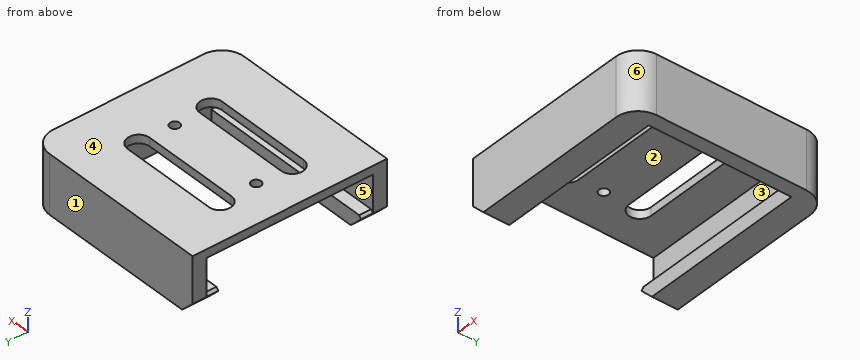
Autodesk Fusion 360 part; units mm, degrees
sketch "Sketch1" plane through (0, 0, 0) normal (0, 0, 1) x (1, 0, 0)
  line L0 (30, 25.7) -> (-30, 25.7)
  line L1 (-30, 25.7) -> (-30, -25.7)
  line L2 (-30, -25.7) -> (30, -25.7)
  line L3 (30, -25.7) -> (30, 25.7)
  line L4 (30, -30) -> (-30, -30)
  line L5 (-30, -35) -> (-30, 35)
  line L6 (-30, 30) -> (30, 30)
  line L7 (30, 30) -> (30, -30)
  line L8 (-30, 35) -> (27, 35)
  line L9 (35, 27) -> (35, -27)
  line L10 (-30, -35) -> (27, -35)
  arc A0 (35, 27) -> (27, 35) centre (27, 27) ccw
  arc A1 (27, -35) -> (35, -27) centre (27, -27) ccw
  circle A2 centre (-20, 0) radius 1.75
  circle A3 centre (15, 0) radius 1.75
  line L11 (-20, 9) -> (15, 9)
  arc A4 (15, 9) -> (15, 17) centre (15, 13) ccw
  line L12 (15, 17) -> (-20, 17)
  arc A5 (-20, 17) -> (-20, 9) centre (-20, 13) ccw
  line L13 (-20, 13) -> (15, 13) construction
  line L14 (1.75, 0) -> (22.5, 0)
  line L15 (-20, -9) -> (15, -9)
  arc A6 (-20, -9) -> (-20, -17) centre (-20, -13) ccw
  line L16 (15, -17) -> (-20, -17)
  arc A7 (15, -17) -> (15, -9) centre (15, -13) ccw
  dimension "d1" = 60
  dimension "d2" = 51.4
  dimension "d3" = 60
  dimension "d6" = 8
  dimension "d15" = 3.5
  dimension "d16" = 3.5
extrude "Extrude1" add sketch "Sketch1" along normal blind 5.5 contours L3 L4 L5 L6 L7 L8 L9 L10 A0 A1 | L0 L5 L6 L7 | L2 L4 L5 L7
extrude "Extrude2" add sketch "Sketch1" along normal blind 18 contours L3 L4 L5 L6 L7 L8 L9 L10 A0 A1
extrude "Extrude3" add sketch "Sketch1" along normal blind 21 and the other way blind -18
sketch "Sketch2" plane through (0, -35, 0) normal (0, -1, 0) x (1, 0, 0)
  line L0 (-30, 0) -> (27, 0)
  line L1 (27, 0) -> (27, 21)
  line L2 (27, 21) -> (-30, 21)
  line L3 (-30, 21) -> (-30, 0)
  line L4 (-30, 0) -> (-34.45, 0)
  line L5 (-34.45, 0) -> (-34.45, 4.55)
  line L6 (-30, 0) -> (-30.316, 0.3196)
  line L7 (-30.316, 0.3196) -> (-34.45, 4.55)
  line L8 (-34.45, 4.55) -> (-34.45, 21)
  line L9 (-34.45, 21) -> (-30, 21)
  line L10 (-30, 0) -> (-30, 5.5)
  line L11 (-30, 5.5) -> (-34.45, 5.5)
  dimension "d17" = 4.45
  dimension "d18" = 4.55
  dimension "d25" = 5.5
extrude "Extrude4" add sketch "Sketch2" against normal blind 5 contours L3 L6 L7 L8 L10 L11 | L3 L8 L9 L11
extrude "Extrude5" add sketch "Sketch2" along normal blind -70 and the other way blind 65 contours L3 L6 L7 L8 L10 L11 | L3 L8 L9 L11
extrude "Extrude6" add sketch "Sketch2" against normal blind 9.3 contours L3 L6 L7 L8 L10 L11
extrude "Extrude7" add sketch "Sketch2" along normal blind -65 and the other way blind 60.7 contours L3 L6 L7 L8 L10 L11
extrude "Extrude8" add 1 faces at (-30, -10, 19) along direction (-1, 0, 0) blind 4.45
chamfer "Chamfer1" distance 0.9 angle 45 2 edges at (-34.45, 27.85, 5.5) (-34.45, -27.85, 5.5)
The model under review builds one solid part; all positions refer to its coordinate system, in mm. Face numbers are marked on the shaded views. A direction names the side the tool comes from. Round coordinates to 2 decimals unless told otherwise and drop trailing zeros. Write each loop counter-clockwise with the first axis right and the second up, starting at its lowest first coordinate (ties: lowest second). Pieces come first, ordered by that corner, then holes. Notation, with made-up numbers: (-33, -1.75) -> (-15, -1.75) arc R26 ccw to (-15, 30.25) -> close; hole circle Ø9 at (-17.75, 56). An arc over 180 degrees is marked (long way). Answer as a JSON object with one key per item and string values.
1. The part is to be moulded in two halves that separate along Y. For the marked faces 3, 4, 5 and 6, say which applies: pulls with the +Y half, pulls with the -Y half, needs draft (parallel to the pull), parting line crosses it, or undercut.
Results found:
{"face 3": "undercut", "face 4": "needs draft", "face 5": "undercut", "face 6": "pulls with the -Y half"}
2. We need section D-D on z = 2.25. State the section outline as (x, y) points.
Results found:
{"outline": "(-32.2, -35) -> (27, -35) arc R8 ccw to (35, -27) -> (35, 27) arc R8 ccw to (27, 35) -> (-32.2, 35) -> (-32.2, 25.7) -> (30, 25.7) -> (30, -25.7) -> (-32.2, -25.7) -> close"}
3. We need section A-A on y = 0. State the section outline as (x, z) points.
Results found:
{"outline": "(-34.45, 18) -> (-21.75, 18) -> (-21.75, 21) -> (-34.45, 21) -> close; (-18.25, 18) -> (13.25, 18) -> (13.25, 21) -> (-18.25, 21) -> close; (16.75, 18) -> (30, 18) -> (30, 0) -> (35, 0) -> (35, 21) -> (16.75, 21) -> close"}
4. We need section C-C on y = -13. State the section outline as (x, z) points.
Results found:
{"outline": "(-34.45, 18) -> (-24, 18) -> (-24, 21) -> (-34.45, 21) -> close; (19, 18) -> (30, 18) -> (30, 0) -> (35, 0) -> (35, 21) -> (19, 21) -> close"}
5. Machinability: for the marked faces 1 and 2, which of the approach directions +Z, -Z, +X, -X, +Y, -Y give a long, thin tool a straight path to every point of the face, cutting with its end or side? Answer none if there is none.
Results found:
{"face 1": "+Z, -Z, +X, -X, +Y", "face 2": "-X"}
6. To check wall thickness, follow line 1 along Y through (x, z) = (15, 19.55); line 2 along Z through (x, y) = (0, -26); line 3 along Y through (x, z) = (9, 6.25). State the ranges of each line that lie inside material, in increasing order.
Results found:
{"line 1": "y = -35 to -17, -9 to -1.75, 1.75 to 9, 17 to 35", "line 2": "z = 0 to 5.5, 18 to 21", "line 3": "y = -35 to -30, 30 to 35"}
7. We need section B-B on x = -16.5. State the section outline as (y, z) points.
Results found:
{"outline": "(-35, 0) -> (-25.7, 0) -> (-25.7, 5.5) -> (-30, 5.5) -> (-30, 18) -> (-17, 18) -> (-17, 21) -> (-35, 21) -> close; (-9, 18) -> (9, 18) -> (9, 21) -> (-9, 21) -> close; (17, 18) -> (30, 18) -> (30, 5.5) -> (25.7, 5.5) -> (25.7, 0) -> (35, 0) -> (35, 21) -> (17, 21) -> close"}
8. Clearance check with flat-ended pins moving along their axes: pin 1 (18 mm diameter, centred on x = 13, y = 4.5, fed in from -Z); pin 2 (3 mm diameter, centred on y = 14, z = 11.5, fed in from -X). State where each tip first meets the part, or that it passes through.
Results found:
{"pin 1": "stops at z = 18", "pin 2": "stops at x = 30"}
